Check sheet for the modelled part. Datum: model origin and axes. Units: mm. Face numbers are marked on the shaded views. Round coordinates to 2 decimals unless told otherwise and drop trailing zeros. Loops run counter-clockwise (first coordinate to the right, second up) from the corner with the lowest first, then second, coordinate; pieces in that order, holes last. Notation, with made-up numbers: (6.25, -26.5) -> (17.25, -26.5) arc R21 cw to (17.25, 8.5) -> close; hole circle Ø2 at (-6, 60). An arc over 180 degrees is marked (long way). Use one line per item in the form item = value. Start each with the question number.
(1) Sectioned sample at C-C (x = -7). Record the cut outline in (y, z).
(2) Material ranges on probe 1 along Z at (x, y) = (5.25, 2.4); probe 2 along X at (y, z) = (1.25, 4.75); probe 3 along X at (y, z) = (4.1, 4), recorded low to high. Write a range as [from, to].
(3) Sectioned sample at D-D (y = 0.35). Record the cut outline in (x, z).
(4) Sectioned sample at B-B (z = -2.54). Record the cut outline in (x, y), and give its area (3 significant figures).
(5) Draft check along X on the marked faces 1, 2, 3 and 4. Enter one of: released by +X, released by -X, zero draft, split by the parting line, or undercut.
(6) Go/stop test with a flat-tipped pin: pin 1 (2.5 mm diameter, centred on x = 1.5, y = 3, fed in from -Z). Record where the tip stops, or that it passes through.
(7) Sectioned sample at A-A (y = 2.54). Record the cut outline in (x, z), and give its area (3 significant figures).
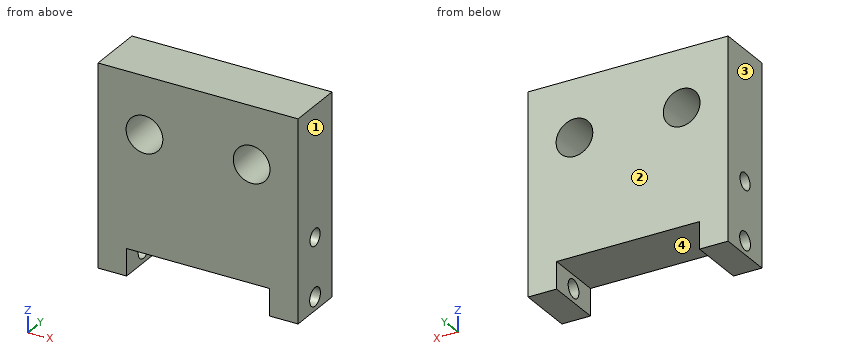
from build123d import *

# Parameters (mm, degrees)
SKETCH1_W             = 17.78
SKETCH1_H             = 17.78
BOSS_EXTRUDE1_DEPTH   = 5.08
SKETCH2_W             = 12.7
SKETCH2_H             = 4.7752
CUT_EXTRUDE1_DEPTH    = 14.55988938
F_4_CLEARANCE_HOLE1_D = 3.2639
F_0_CLEARANCE_HOLE1_D = 1.6129
F_1_72_TAPPED_HOLE1_D = 1.5113


with BuildPart() as part:
    # Sketch1 → Boss-Extrude1 (new body)
    with BuildSketch(Plane(origin=(0, 0, 0), x_dir=(1, 0, 0), z_dir=(0, 1, 0))):
        Rectangle(SKETCH1_W, SKETCH1_H)
    extrude(amount=BOSS_EXTRUDE1_DEPTH)

    # Sketch2 → Cut-Extrude1 (cut, through all)
    with BuildSketch(Plane(origin=(0, 5.08, 0), x_dir=(1, 0, 0), z_dir=(0, 1, 0))):
        with Locations((0, 8.89)):
            Rectangle(SKETCH2_W, SKETCH2_H)
    extrude(amount=-CUT_EXTRUDE1_DEPTH, mode=Mode.SUBTRACT)

    # #4 Clearance Hole1 (through all)
    with Locations(Plane(origin=(0, 5.08, 0), x_dir=(1, 0, 0), z_dir=(0, 1, 0))):
        with Locations((4.7625, -3.81), (-4.7625, -3.81)):
            Hole(F_4_CLEARANCE_HOLE1_D / 2)

    # #0 Clearance Hole1 (through all)
    with Locations(Plane(origin=(8.89, 0, 0), x_dir=(0, 0, -1), z_dir=(1, 0, 0))):
        with Locations((7.6962, 2.54)):
            Hole(F_0_CLEARANCE_HOLE1_D / 2)

    # #1-72 Tapped Hole1 (through all)
    with Locations(Plane(origin=(8.89, 0, 0), x_dir=(0, 0, -1), z_dir=(1, 0, 0))):
        with Locations((2.54, 2.54)):
            Hole(F_1_72_TAPPED_HOLE1_D / 2)


solid = part.part
Checks:
q1.outline = (0, -8.89) -> (5.08, -8.89) -> (5.08, 8.89) -> (0, 8.89) -> close; hole circle Ø1.61 at (2.54, -7.7); hole circle Ø1.51 at (2.54, -2.54)
q2.probe_1 = [-6.5, -3.28], [-1.8, 2.25], [5.37, 8.89]
q2.probe_2 = [-8.89, -6.1], [-3.43, 3.43], [6.1, 8.89]
q2.probe_3 = [-8.89, -6.38], [-3.14, 3.14], [6.38, 8.89]
q3.outline = (-8.89, -8.89) -> (-6.35, -8.89) -> (-6.35, -6.5) -> (6.35, -6.5) -> (6.35, -8.89) -> (8.89, -8.89) -> (8.89, 8.89) -> (-8.89, 8.89) -> close; hole circle Ø3.26 at (-4.76, 3.81); hole circle Ø3.26 at (4.76, 3.81)
q4.outline = (-8.89, 0) -> (8.89, 0) -> (8.89, 1.78) -> (-8.89, 1.78) -> close; (-8.89, 3.3) -> (8.89, 3.3) -> (8.89, 5.08) -> (-8.89, 5.08) -> close
q4.area = 63.5 mm2
q5.face_1 = released by +X
q5.face_2 = zero draft
q5.face_3 = released by -X
q5.face_4 = undercut
q6.pin_1 = -6.5
q7.outline = (-8.89, -8.89) -> (-6.35, -8.89) -> (-6.35, -8.5) -> (-8.89, -8.5) -> close; (-8.89, -6.89) -> (-6.35, -6.89) -> (-6.35, -6.5) -> (6.35, -6.5) -> (6.35, -6.89) -> (8.89, -6.89) -> (8.89, -3.3) -> (-8.89, -3.3) -> close; (-8.89, -1.78) -> (8.89, -1.78) -> (8.89, 8.89) -> (-8.89, 8.89) -> close; (6.35, -8.89) -> (8.89, -8.89) -> (8.89, -8.5) -> (6.35, -8.5) -> close; hole circle Ø3.26 at (-4.76, 3.81); hole circle Ø3.26 at (4.76, 3.81)
q7.area = 234 mm2
